Answer from the drawing. Dimensions are ordinates in mm from the lowest x, y and z of the part. A direction names the side the tool comes from. Round coordinates to 2 decimals unless told otherwise and drop trailing zeros. Order: outer loops, then holes, each group sorted by start corner. A loop starts at its lowest first (then second) coordinate and runs counter-clockwise, first axis right, second up. Notation, with made-up numbers: M -3,69 L 47,69 A24 ccw 47,82 Z; hole C 29,65 d6. An arc over 180 degrees is marked long. Write item = value, one per line. Start each with the question number.
(1) A cutting plane is placed at C-C, the plane y = 33. Determine the outline of the cut face in (x, z) (1 decimal), and give its area (3 significant figures).
(2) A cutting plane is placed at B-B, the plane z = 12.7. Determine the outline of the cut face in (x, y) (1 decimal), and give its area (3 significant figures).
(3) Which of the six approach directions +Z, -Z, +X, -X, +Y, -Y give full straight-line access (tool end or side, diameter ignored) to the marked faces 1 and 2?
(4) Each of these flat-tipped pins is pushed along its axis until it touches: pin 1 (4 mm diameter, centred on x = 37.5, z = 12, fed in from -Y) (3 decimals); pin 2 (8 mm diameter, centred on x = 10.5, y = 16.5, fed in from +Z). Where does it stop, or does it pass through?
(5) Straight lines are drawn through the part: probe 1 along Z at (x, y) = (50.8, 49.5); probe 2 along X at (y, z) = (49.6, 63.5); probe 3 along X at (y, z) = (4, 15) (1 decimal). For each, find the intervals that lie inside material, in ascending order. Write a range as from..to.
(6) A cutting plane is placed at D-D, the plane z = 24.5. Determine the outline of the cut face in (x, y) (1 decimal), and give its area (3 significant figures).
(7) A cutting plane is placed at A-A, the plane x = 12.7. Determine the outline of the cut face in (y, z) (1 decimal), and give its area (3 significant figures).
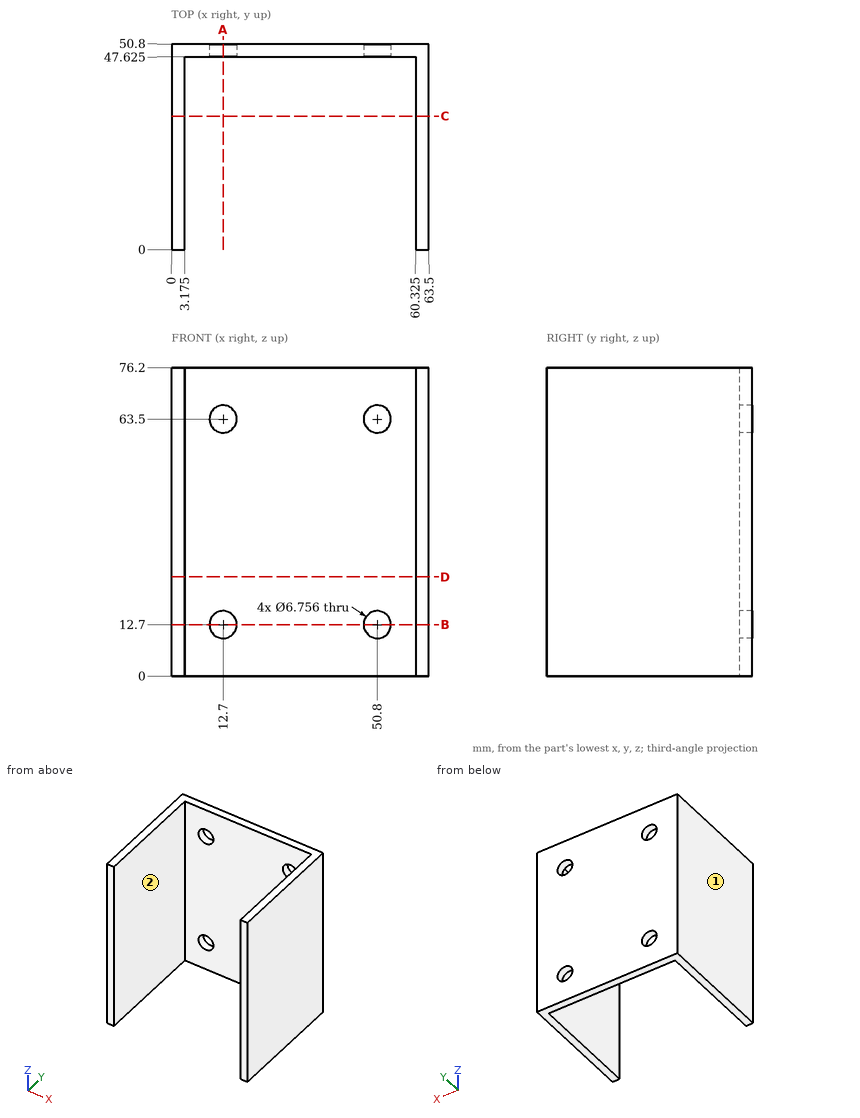
Reported:
q1.outline = M 0,0 L 3.2,0 L 3.2,76.2 L 0,76.2 Z; M 60.3,0 L 63.5,0 L 63.5,76.2 L 60.3,76.2 Z
q1.area = 484 mm²
q2.outline = M 0,0 L 3.2,0 L 3.2,47.6 L 9.3,47.6 L 9.3,50.8 L 0,50.8 Z; M 16.1,47.6 L 47.4,47.6 L 47.4,50.8 L 16.1,50.8 Z; M 54.2,47.6 L 60.3,47.6 L 60.3,0 L 63.5,0 L 63.5,50.8 L 54.2,50.8 Z
q2.area = 461 mm²
q3.face_1 = +Z, -Z, -X, +Y, -Y
q3.face_2 = +Z, -Z, -Y
q4.pin_1 = 47.625
q4.pin_2 = through
q5.probe_1 = 0..9.32, 16.08..60.12, 66.88..76.2
q5.probe_2 = 0..9.32, 16.08..47.42, 54.18..63.5
q5.probe_3 = 0..3.2, 60.3..63.5
q6.outline = M 0,0 L 3.2,0 L 3.2,47.6 L 60.3,47.6 L 60.3,0 L 63.5,0 L 63.5,50.8 L 0,50.8 Z
q6.area = 504 mm²
q7.outline = M 47.6,0 L 50.8,0 L 50.8,9.3 L 47.6,9.3 Z; M 47.6,16.1 L 50.8,16.1 L 50.8,60.1 L 47.6,60.1 Z; M 47.6,66.9 L 50.8,66.9 L 50.8,76.2 L 47.6,76.2 Z
q7.area = 199 mm²
